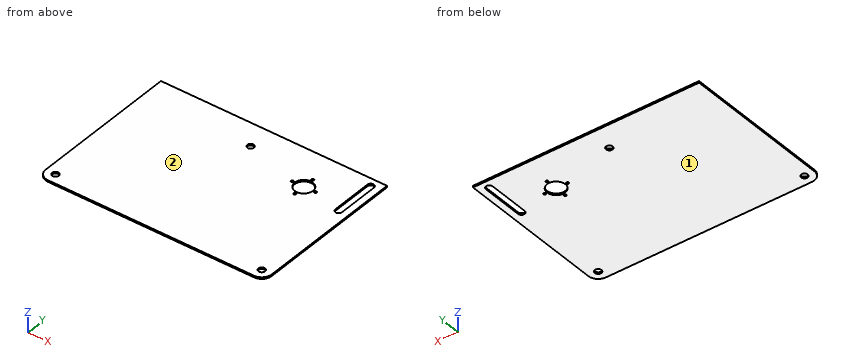
```python
from build123d import *

# Parameters (mm, degrees)
SKETCH1_R           = 4
SKETCH1_R_2         = 1.5
SKETCH1_R_3         = 11
BOSS_EXTRUDE1_DEPTH = 2


with BuildPart() as part:
    # Sketch1 → Boss-Extrude1 (new body)
    with BuildSketch(Plane.XY):
        with BuildLine():
            ThreePointArc((-137, 0), (-133.485281374, -8.485281374), (-125, -12))
            Line((-125, -12), (125, -12))
            ThreePointArc((125, -12), (133.485281374, -8.485281374), (137, 0))
            Line((137, 0), (137, 180))
            Line((137, 180), (-53.998245329, 180))
            Line((-53.998245329, 180), (-137, 180))
            Line((-137, 180), (-137, 0))
        make_face()
        with Locations((-125, 0)):
            Circle(SKETCH1_R, mode=Mode.SUBTRACT)
        with Locations((125, 0)):
            Circle(SKETCH1_R, mode=Mode.SUBTRACT)
        with Locations((-5, 150)):
            Circle(SKETCH1_R, mode=Mode.SUBTRACT)
        with Locations((61, 130)):
            Circle(SKETCH1_R_2, mode=Mode.SUBTRACT)
        with Locations((75, 116)):
            Circle(SKETCH1_R_2, mode=Mode.SUBTRACT)
        with Locations((75, 130)):
            Circle(SKETCH1_R_3, mode=Mode.SUBTRACT)
        with Locations((89, 130)):
            Circle(SKETCH1_R_2, mode=Mode.SUBTRACT)
        with Locations((75, 144)):
            Circle(SKETCH1_R_2, mode=Mode.SUBTRACT)
        with BuildLine():
            ThreePointArc((129, 120), (125, 116), (121, 120))
            Line((121, 120), (121, 170))
            ThreePointArc((121, 170), (125, 174), (129, 170))
            Line((129, 170), (129, 120))
        make_face(mode=Mode.SUBTRACT)
    extrude(amount=BOSS_EXTRUDE1_DEPTH)


solid = part.part
```
Input: part model. Units: mm. Frame: model coordinates. Face numbers are marked on the shaded views. Coordinates: 2 decimals unless noted, no trailing zeros. Order: outer loops, then holes, each group sorted by start corner. A loop starts at its lowest first (then second) coordinate and runs counter-clockwise, first axis right, second up. Notation, with made-up numbers: (46.5, -27) - (52.5, -27) arc R12 ccw to (52.5, -9) - close; hole circle Ø8 at (-14, -9.5). An arc over 180 degrees is marked (long way). Return JSON: item names as keys, results as strings.
Q1. Cut plane A-A (z = 1.25). State how many separate pieces and enclosed holes the cut face has, then the cut area to 3 significant figures.
The answers:
{"separate pieces": "1", "enclosed holes": "9", "area": "51,500 mm2"}
Q2. Cut plane B-B (y = 150). Return loops of the section in (x, z).
The answers:
{"outline": "(-137, 0) - (-9, 0) - (-9, 2) - (-137, 2) - close; (-1, 0) - (121, 0) - (121, 2) - (-1, 2) - close; (129, 0) - (137, 0) - (137, 2) - (129, 2) - close"}
Q3. Ray query, probe 1 along Y at (x, z) = (75, 0.4); probe 2 along X at (y, z) = (144, 1.6); probe 3 along Y at (x, z) = (61, 0.7). Return the intervals inside material, ascending.
The answers:
{"probe 1": "y = -12 to 114.5, 117.5 to 119, 141 to 142.5, 145.5 to 180", "probe 2": "x = -137 to 73.5, 76.5 to 121, 129 to 137", "probe 3": "y = -12 to 128.5, 131.5 to 180"}
Q4. Draft query along Z for the marked faces 1 and 2. Return one class per face: +Z half, -Z half, draft (parallel to the pull), parting line (faces both ways), or undercut.
The answers:
{"face 1": "-Z half", "face 2": "+Z half"}
Q5. First-contact query: pin 1 (6.5 mm diameter, centred on x = 125, y = 0, fed in from +Z). Flat tip, straight axial feed; report the tip coordinate or a pass-through.
The answers:
{"pin 1": "passes through"}
